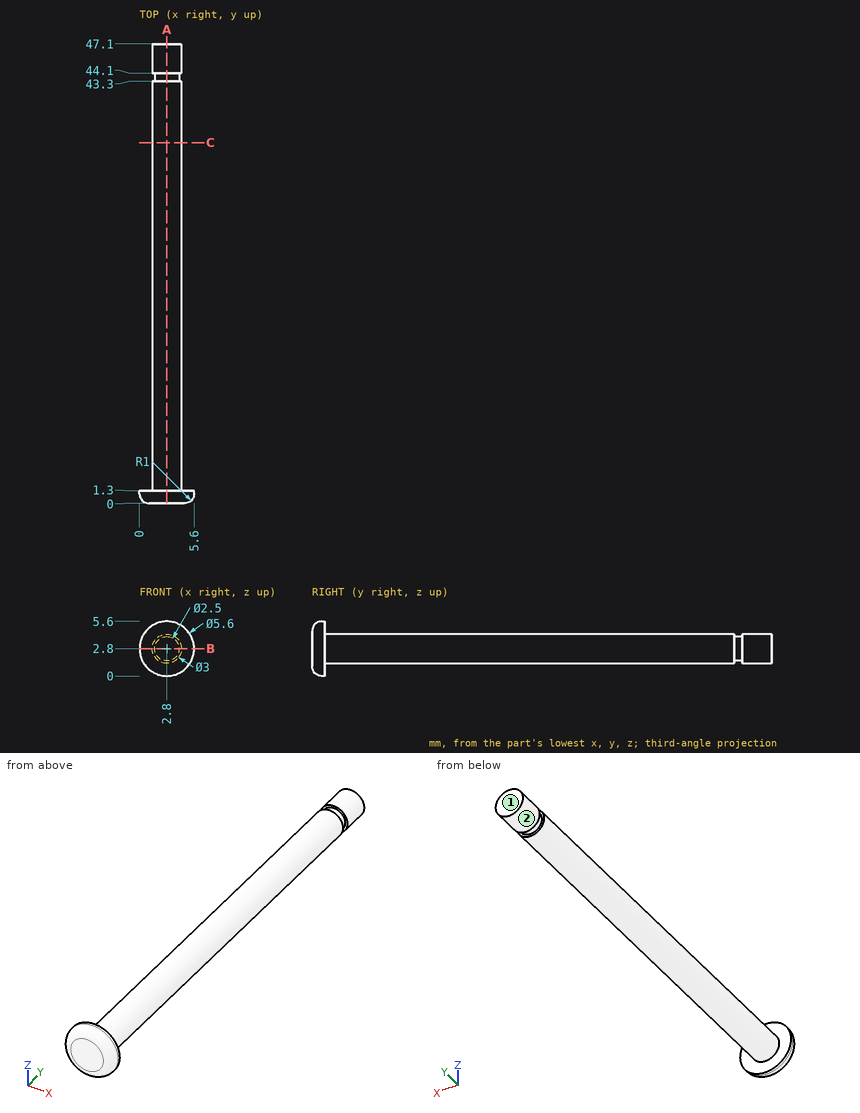
Verification items for this drawing (mm, ordinates from the low corner). A direction names the side the tool comes from. Give positions to 0.01 mm unless a question says otherwise; leave off trailing zeros. Write each loop counter-clockwise with the first axis right and the second up, starting at its lowest first coordinate (ties: lowest second). Pieces come first, ordered by that corner, then holes. Notation, with made-up numbers: (-21, 56.25) - (6, 56.25) arc R27 cw to (6, 78.25) - close; hole circle Ø5 at (60, 46.5). An arc over 180 degrees is marked (long way). Answer as CSV lines item,"result". Start each with the question number.
1. Sectioned sample at A-A (x = 2.8). Record the boundary of the cut face in (y, z), then the cut area to 3 significant figures.
2. Depth check by flat-ended pin: pin 1 (1.5 mm diameter, centred on x = 1, y = 16, fed in from +Z); pin 2 (1.5 mm diameter, centred on x = 2, z = 2.5, fed in from -Y); pin 3 (2 mm diameter, centred on y = 18, z = 3, fed in from +X). Enter the tip coordinate at first touch or a pass-through.
3. Sectioned sample at B-B (z = 2.8). Record the boundary of the cut face in (x, y), then the cut area to 3 significant figures.
4. Set-up check for the marked faces 1 and 2: record each of +Z, -Z, +X, -X, +Y, -Y from which the full face is reachable in a straight line by a thin tool's end or side.
5. Sectioned sample at C-C (y = 37). Record the boundary of the cut face in (x, z).
6. Thickness scan on line 1 (Z direction, x = 2.65, y = 25); line 2 (Y direction, x = 4.2, z = 3.9); line 3 (Y direction, x = 2.15, z = 3.9). Record the ranges inside material, lowest first.
Derived:
1,outline,"(0, 1) arc R1 ccw to (1, 0) - (1.3, 0) - (1.3, 1.3) - (43.3, 1.3) - (43.3, 1.55) - (44.1, 1.55) - (44.1, 1.3) - (47.1, 1.3) - (47.1, 4.3) - (44.1, 4.3) - (44.1, 4.05) - (43.3, 4.05) - (43.3, 4.3) - (1.3, 4.3) - (1.3, 5.6) - (1, 5.6) arc R1 ccw to (0, 4.6) - close"
1,area,"144 mm²"
2,pin 1,"z = 3.87"
2,pin 2,"y = 0"
2,pin 3,"x = 4.3"
3,outline,"(0, 1) arc R1 ccw to (1, 0) - (4.6, 0) arc R1 ccw to (5.6, 1) - (5.6, 1.3) - (4.3, 1.3) - (4.3, 43.3) - (4.05, 43.3) - (4.05, 44.1) - (4.3, 44.1) - (4.3, 47.1) - (1.3, 47.1) - (1.3, 44.1) - (1.55, 44.1) - (1.55, 43.3) - (1.3, 43.3) - (1.3, 1.3) - (0, 1.3) - close"
3,area,"144 mm²"
4,face 1,"+Z, -Z, +X, -X, +Y"
4,face 2,"+Y"
5,outline,"circle Ø3 at (2.8, 2.8)"
6,line 1,"1.31 to 4.29"
6,line 2,"0 to 1.3"
6,line 3,"0 to 43.3, 44.1 to 47.1"
